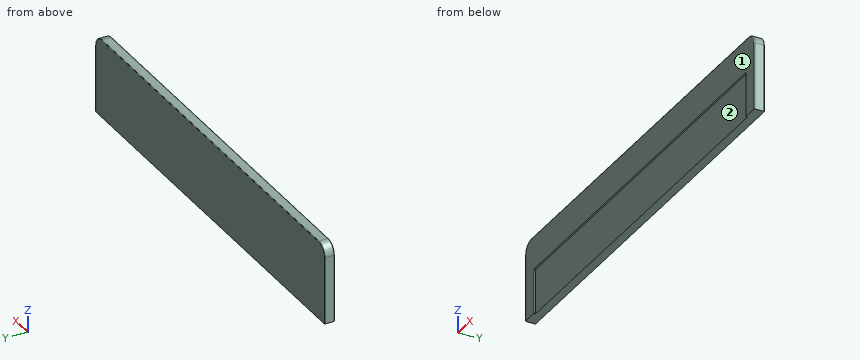
```python
from build123d import *

# Parameters (mm, degrees)
F1_DEPTH = 9
F0_W     = 173
F0_H     = 40
F2_DEPTH = 7.5
F3_R     = 10
F4_R     = 1
F5_R     = 0.5


with BuildPart() as f1:
    # F0 (on Front) → F1 (new body)
    with BuildSketch(Plane.XZ):
        Polygon((137.2830025838, 31.1808919907), (-49.7169974162, 31.1808919907), (-49.7169974162, -38.8191080093), (-35.7169974162, -38.8191080093), (-35.7169974162, 1.1808919907), (137.2830025838, 1.1808919907), align=None)
    extrude(amount=F1_DEPTH)

    # F0 (on Front) → F2 (join)
    with BuildSketch(Plane.XZ):
        Polygon((137.2830025838, 31.1808919907), (-49.7169974162, 31.1808919907), (-49.7169974162, -38.8191080093), (-35.7169974162, -38.8191080093), (-35.7169974162, 1.1808919907), (137.2830025838, 1.1808919907), align=None)
        with Locations((50.7830025838, -18.8191080093)):
            Rectangle(F0_W, F0_H)
    extrude(amount=F2_DEPTH)

    # F3
    f3_edges = [f1.edges().sort_by_distance(p)[0] for p in [
        (-49.716997, -4.5, 31.180892),
    ]]
    fillet(f3_edges, radius=F3_R)

    # F4
    f4_edges = [f1.edges().sort_by_distance(p)[0] for p in [
        (48.783003, -9, 31.180892),
        (-46.788065, -9, 28.25196),
        (-49.716997, -9, -8.819108),
    ]]
    fillet(f4_edges, radius=F4_R)

    # F5
    f5_edges = [f1.edges().sort_by_distance(p)[0] for p in [
        (48.783003, 0, 31.180892),
        (-46.788065, 0, 28.25196),
        (-49.716997, 0, -8.819108),
    ]]
    fillet(f5_edges, radius=F5_R)

    # F6: F1 across face


with BuildPart() as f1_1:
    add(f1.part)
    add(f1.part.mirror(Plane(origin=(137.2830025838, -4.1038796524, -2.2558019442), x_dir=(0, 1, 0), z_dir=(1, 0, 0))))


solid = f1_1.part
```
Could you check a few things on this model? Use its own coordinates, in mm. Face numbers are marked on the shaded views. Round coordinates to 2 decimals unless told otherwise and drop trailing zeros. Loops run counter-clockwise (first coordinate to the right, second up) from the corner with the lowest first, then second, coordinate; pieces in that order, holes last.
Q1. Thinking about a two-plate mould opening in X: for the marked faces 1 and 2, which applies, pulls with the +X half, pulls with the -X half, needs draft (parallel to the pull), parting line crosses it, or undercut?
Q2. I want a section at B-B (x = 6). Write out the boundary of the cut face in (y, z), and give its area (3 significant figures).
Q3. I want a section at A-A (z = -10). Write out the boundary of the cut face in (x, y), and give its area (3 significant figures).
Q4. Please list where these lines run through material, in increasing order: L1, parallel to Y at x = 30.5, z = 0.5; L2, parallel to Z at x = 294.5, y = -8; L3, parallel to Z at x = 139, y = -0.25.
Q5. For P1, Ø3, axis at x = 95, z = -9, coming from the -Y side; P2, Ø0.8, axis at y = -8.5, z = -9, coming from the -X side; P3, Ø0.8, axis at x = 82.5, y = -8, coming from the -Z side, each with a flat end and sliding along its axis, tell me the tip position at first contact or that it passes through.
Answer below:
1. face 1: needs draft
1. face 2: undercut
2. outline: (-9, 1.18) - (-7.5, 1.18) - (-7.5, -38.82) - (0, -38.82) - (0, 30.68) arc R0.5 ccw to (-0.5, 31.18) - (-8, 31.18) arc R1 ccw to (-9, 30.18) - close
2. area: 570 mm2
3. outline: (-49.72, -8) arc R1 ccw to (-48.72, -9) - (-35.72, -9) - (-35.72, -7.5) - (310.28, -7.5) - (310.28, -9) - (323.28, -9) arc R1 ccw to (324.28, -8) - (324.28, -0.5) arc R0.5 ccw to (323.78, 0) - (-49.22, 0) arc R0.5 ccw to (-49.72, -0.5) - close
3. area: 2,850 mm2
4. L1: y = -7.5 to 0
4. L2: z = 1.18 to 31.18
4. L3: z = -38.82 to 31.11
5. P1: stops at y = -7.5
5. P2: stops at x = -49.71
5. P3: stops at z = 1.18
